Can you work these out from the model? Positions are in its coordinate system, mm. Give positions to 0.01 mm unless a question says otherwise; leave off trailing zeros. Order: outer loops, then holes, each group sorted by start corner. A loop starts at its lowest first (then second) coordinate and runs counter-clockwise, first axis right, second up. Notation, with made-up numbers: (74, 59.25) - (120, 59.25) arc R12 ccw to (120, 66.25) - close; hole circle Ø4 at (20, 37.5). An arc over 180 degrees is marked (long way). Return JSON: item names as keys, results as strings.
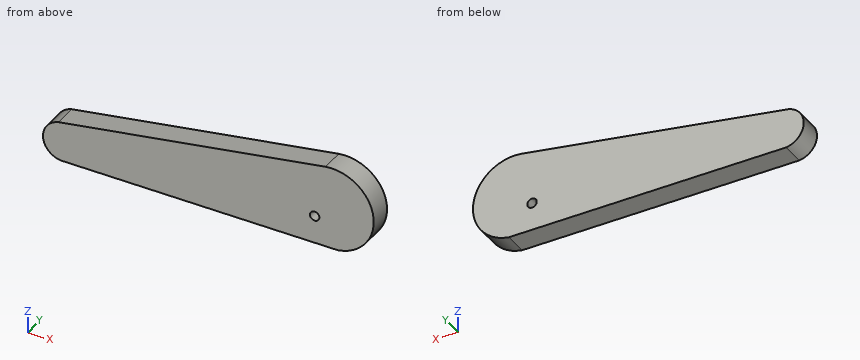
```python
from build123d import *

# Parameters (mm, degrees)
F1_DEPTH = 8.73125
F2_R     = 1.7859375
F3_DEPTH = 8.73125


# Not quite as in the source:
# - a length typed as a fraction of an inch, garbled in the dataset ("3 / 203.2 mm" for 3/8 in), is restored


with BuildPart() as f1:
    # F0 (on Front) → F1 (new body)
    with BuildSketch(Plane.XZ):
        with BuildLine():
            Line((16.3863981424, 24.04380231), (-84.6225991332, 7.4210920542))
            ThreePointArc((-84.6225991332, 7.4210920542), (-90.4179458573, -0.3797760525), (-83.7262291187, -7.42679769))
            Line((-83.7262291187, -7.42679769), (21.0487708813, -7.42679769))
            ThreePointArc((21.0487708813, -7.42679769), (34.4528845118, 10.6396886794), (16.3863981424, 24.04380231))
        make_face()
    extrude(amount=F1_DEPTH)

    # F2 (on face) → F3 (cut, through all)
    with BuildSketch(Plane.XZ.offset(8.73125)):
        with Locations((12.2811356559, 3.1172726303)):
            Circle(F2_R)
    extrude(amount=-F3_DEPTH, mode=Mode.SUBTRACT)


solid = f1.part
```
1. Suppose I cut it at A-A (y = -4.75). List the corners of the cut face in (x, z) for me.
Checks:
{"outline": "(-84.62, 7.42) arc R7.55 ccw to (-83.73, -7.43) - (21.05, -7.43) arc R15.91 ccw to (16.39, 24.04) - close; hole circle Ø3.57 at (12.28, 3.12)"}
2. Suppose I cut it at C-C (x = -14). List the corners of the cut face in (y, z) for me, plus the area to 3 significant figures.
Checks:
{"outline": "(-8.73, -7.43) - (0, -7.43) - (0, 19.04) - (-8.73, 19.04) - close", "area": "231 mm^2"}
3. Suppose I cut it at B-B (z = 9.5). List the corners of the cut face in (x, y) for me, plus the area to 3 significant figures.
Checks:
{"outline": "(-71.99, -8.73) - (34.58, -8.73) - (34.58, 0) - (-71.99, 0) - close", "area": "930 mm^2"}
4. If I drill on L1, parallel to X at y = -6.25, z = 2.5; L2, parallel to X at y = -5.75, z = 1.5; L3, parallel to Z at x = -67, y = -5, over which ranges is the centre line in solid material (lowest first)? Write a range as [from, to].
Checks:
{"L1": "[-90.03, 10.61], [13.96, 33.53]", "L2": "[-90.3, 11.52], [13.04, 33.09]", "L3": "[-7.43, 10.32]"}
5. For pin 1 Ø1.5 at (x, y) = (-50, -4) entering from +Z; pin 2 Ø1.5 at (x, y) = (-63, -3.5) entering from +Z; pin 3 Ø2 at (y, z) = (-4.5, 3.5) entering from +X, each with a flat end and sliding along its axis, tell me the tip position at first contact or that it passes through.
Checks:
{"pin 1": "z = 13.24", "pin 2": "z = 11.1", "pin 3": "x = 34.16"}
